Input: dimensioned drawing with shaded views. Units: mm. Origin: part minimum x, y, z. A direction names the side the tool comes from. Give positions to 0.01 mm unless a question says otherwise; leave off trailing zeros. Write each loop counter-clockwise with the first axis right and the second up, starting at its lowest first coordinate (ties: lowest second). Pieces come first, ordered by that corner, then holes. Notation, with made-up numbers: (27, -37) - (46, -37) arc R33 cw to (46, -2) - close; hole circle Ø5 at (83, 53). An arc over 180 degrees is marked (long way). Answer as a JSON object with one key per item and string values. Group by question number.
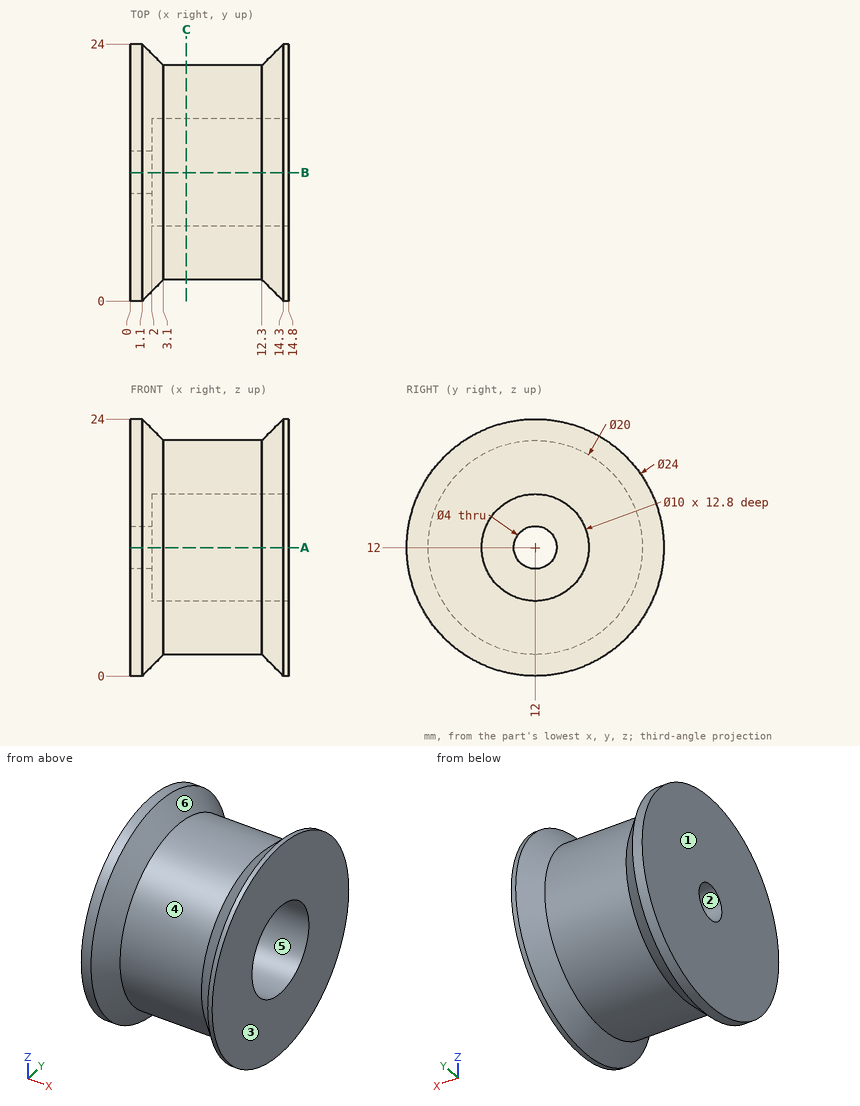
1) Cut plane A-A on z = 12. Return the cut outline in (x, y), and give its area (3 significant figures).
2) Reachability of the marked faces 5 and 6 from +Z, -Z, +X, -X, +Y, -Y: full face, straight path, thin tool, end or side. Return the list, or none.
3) Cut plane C-C on x = 5.25. Return the cut outline in (y, z), and give its area (3 significant figures).
4) Mould query, pull axis X, two halves, no side actions, for the marked faces 1, 2, 3 and 4. Classes: +X half, -X half, draft (parallel to the pull), parting line (faces both ways), or undercut.
5) Pin query (flat end, axial travel): P1, Ø11, axis at y = 13.5, z = 14, coming from the +X side; P2, Ø6, axis at y = 12, z = 12, coming from the +X side; P3, Ø4, axis at x = 6.5, z = 5, coming from the -Y side; P4, Ø2, axis at x = 5.5, z = 11.5, coming from the +Y side. Return the tip coordinate at first contact, or that it passes through.
6) Line query: line 1 along Y through (x, z) = (0.4, 12); line 2 along X through (y, z) = (16, 9.75); line 3 along Y through (x, z) = (6.5, 12.5). Output: solid intervals per line, ascending. Write a range as from..to.
Filled in:
{
 "1": {"outline": "(0, 0) - (1.1, 0) - (3.1, 2) - (12.3, 2) - (14.3, 0) - (14.8, 0) - (14.8, 7) - (2, 7) - (2, 10) - (0, 10) - close; (0, 14) - (2, 14) - (2, 17) - (14.8, 17) - (14.8, 24) - (14.3, 24) - (12.3, 22) - (3.1, 22) - (1.1, 24) - (0, 24) - close", "area": "174 mm²"},
 "2": {"face 5": "+X", "face 6": "none"},
 "3": {"outline": "circle Ø20 at (12, 12); hole circle Ø10 at (12, 12)", "area": "236 mm²"},
 "4": {"face 1": "-X half", "face 2": "draft", "face 3": "+X half", "face 4": "undercut"},
 "5": {"P1": "stops at x = 14.8", "P2": "stops at x = 2", "P3": "stops at y = 3.34", "P4": "stops at y = 22"},
 "6": {"line 1": "y = 0..10, 14..24", "line 2": "x = 0..2", "line 3": "y = 2.01..7.03, 16.97..21.99"}
}
